For this review, take the finished solid that the model builds, in its own axes (mm). Coordinates: 2 decimals unless noted, no trailing zeros. Order: outer loops, then holes, each group sorted by start corner. A loop starts at its lowest first (then second) coordinate and runs counter-clockwise, first axis right, second up. Notation, with made-up numbers: (36, 10.5) - (43, 10.5) arc R4 cw to (43, 16.5) - close; hole circle Ø7 at (-7, -5.5). An arc over 180 degrees is marked (long way). One line per item, written item: value. Start each with the question number.
(1) To check wall thickness, follow line 1 along X through (y, z) = (51, 38.5); line 2 along Y through (x, z) = (-93.5, 23); line 3 along Z through (x, y) = (-43.5, 39). State the ranges of each line that lie inside material, in increasing order.
(2) Consider section C-C on x = -20.5. Write out the cut boundary in (y, z).
(3) Consider section A-A on y = 59. Write out the cut boundary in (x, z).
(4) Clearance check with flat-ended pins moving along their axes: pin 1 (1.5 mm diameter, centred on x = -21, y = 79.5, fed in from -Z); pin 2 (3 mm diameter, centred on x = -89, z = 57, fed in from -Y); pin 3 (5 mm diameter, centred on x = -81, y = 37, fed in from +Z); pin 4 (10 mm diameter, centred on x = -39.5, z = 29, fed in from +Y). State where each tip first meets the part, or that it passes through.
(5) Consider section B-B on z = 45.5. Write out the cut boundary in (x, y).
```python
from build123d import *

# Parameters (mm, degrees)
F0_W     = 110
F0_H     = 120
F1_DEPTH = 72
F3_DEPTH = 120
F5_DEPTH = 133
F7_DEPTH = 133


with BuildPart() as f1:
    # F0 (on Top) → F1 (new body)
    with BuildSketch(Plane.XY):
        with Locations((-55, 60)):
            Rectangle(F0_W, F0_H)
    extrude(amount=F1_DEPTH)

    # F2 (on face) → F3 (cut)
    with BuildSketch(Plane.XZ):
        Polygon((-26.205857, 72), (0, 0), (0, 72), align=None)
    extrude(amount=-F3_DEPTH, mode=Mode.SUBTRACT)

    # F4 (on Right) → F5 (cut)
    with BuildSketch(Plane.YZ):
        Polygon((120, 0), (120, 72), (93.794143, 72), align=None)
    extrude(amount=-F5_DEPTH, mode=Mode.SUBTRACT)

    # F6 (on Right) → F7 (cut)
    with BuildSketch(Plane.YZ):
        Polygon((0, 28.263073), (93.794143, 72), (0, 72), align=None)
    extrude(amount=-F7_DEPTH, mode=Mode.SUBTRACT)


solid = f1.part
```
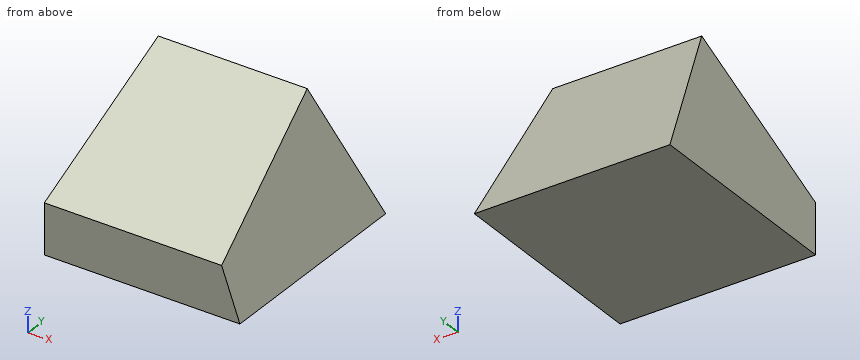
Geometry check:
1. line 1: x = -110 to -14.01
1. line 2: y = 0 to 111.63
1. line 3: z = 0 to 46.45
2. outline: (0, 0) - (120, 0) - (99.5, 56.32) - (60.18, 56.32) - (0, 28.26) - close
3. outline: (-110, 0) - (0, 0) - (-20.3, 55.78) - (-110, 55.78) - close
4. pin 1: stops at z = 0
4. pin 2: stops at y = 58.41
4. pin 3: stops at z = 46.68
4. pin 4: stops at y = 111.26
5. outline: (-110, 36.96) - (-16.56, 36.96) - (-16.56, 103.44) - (-110, 103.44) - close
